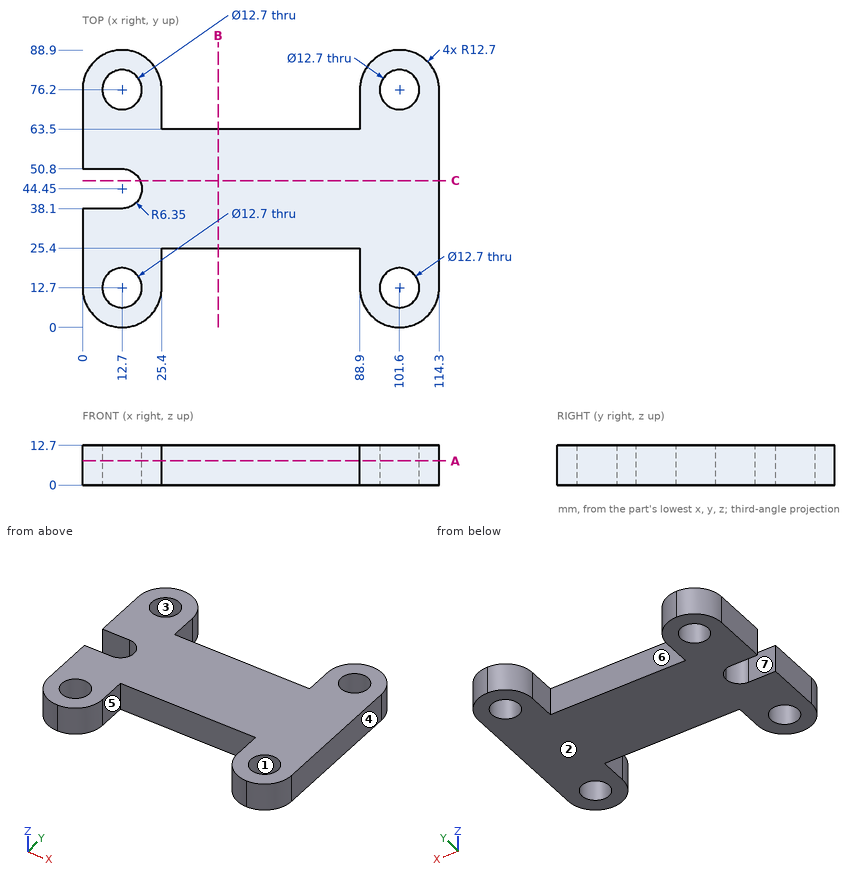
Part print with two shaded views. Sizes in mm from the minimum x, y, z corner. A direction names the side the tool comes from. Round coordinates to 2 decimals unless told otherwise and drop trailing zeros. Write each loop counter-clockwise with the first axis right and the second up, starting at its lowest first coordinate (ties: lowest second). Pieces come first, ordered by that corner, then holes. Notation, with made-up numbers: (-4, -31.75) -> (10, -31.75) arc R29 ccw to (10, -3.75) -> close; hole circle Ø1 at (1.25, 61). An arc over 180 degrees is marked (long way). Use one line per item in the form item = value.
Q1. Drill centre lines: L1, parallel to X at y = 68, z = 5; L2, parallel to Y at x = 51, z = 6.5; L3, parallel to Y at x = 16.5, z = 11.5. Where is each one in solid material? Low to high.
Conclusion:
L1 = 0 to 25.4, 88.9 to 114.3
L2 = 25.4 to 63.5
L3 = 0.58 to 7.61, 17.79 to 39.36, 49.54 to 71.11, 81.29 to 88.32
Q2. Band-saw the part on A-A, the plane z = 7.75. Write the cut outline in (x, y).
Conclusion:
outline = (0, 12.7) arc R12.7 ccw to (25.4, 12.7) -> (25.4, 25.4) -> (88.9, 25.4) -> (88.9, 12.7) arc R12.7 ccw to (114.3, 12.7) -> (114.3, 76.2) arc R12.7 ccw to (88.9, 76.2) -> (88.9, 63.5) -> (25.4, 63.5) -> (25.4, 76.2) arc R12.7 ccw to (0, 76.2) -> (0, 50.8) -> (12.7, 50.8) arc R6.35 cw to (12.7, 38.1) -> (0, 38.1) -> close; hole circle Ø12.7 at (12.7, 12.7); hole circle Ø12.7 at (12.7, 76.2); hole circle Ø12.7 at (101.6, 12.7); hole circle Ø12.7 at (101.6, 76.2)
Q3. Band-saw the part on B-B, the plane x = 43.5. Write the cut outline in (y, z), then the cut area to 3 significant figures.
Conclusion:
outline = (25.4, 0) -> (63.5, 0) -> (63.5, 12.7) -> (25.4, 12.7) -> close
area = 484 mm²
Q4. Drop flat-ended pins along their axis: P1, Ø4, axis at x = 9, z = 4, coming from the -Y side; P2, Ø4, axis at x = 71, z = 3, coming from the -Y side; P3, Ø2, axis at x = 20, z = 2.5, coming from the +Y side. Give the stop position or say it passes through.
Conclusion:
P1 = 0.11
P2 = 25.4
P3 = 87.23
Q5. Band-saw the part on C-C, the plane y = 47. Write the cut outline in (x, z), then the cut area to 3 significant figures.
Conclusion:
outline = (18.52, 0) -> (114.3, 0) -> (114.3, 12.7) -> (18.52, 12.7) -> close
area = 1,220 mm²
Q6. Two-plate mould, pull along X, no slides. Class the marked faces 1, 2, 3 and 4: released by +X, released by -X, zero draft, split by the parting line, or undercut.
Conclusion:
face_1 = undercut
face_2 = zero draft
face_3 = undercut
face_4 = released by +X
Q7. Tool access for the marked faces 5, 6 and 7: list every direction of +Z, -Z, +X, -X, +Y, -Y with a clear straight run to the whole face (end or side of a thin tool).
Conclusion:
face_5 = +Z, -Z, -Y
face_6 = +Z, -Z, +Y
face_7 = +Z, -Z, -X
